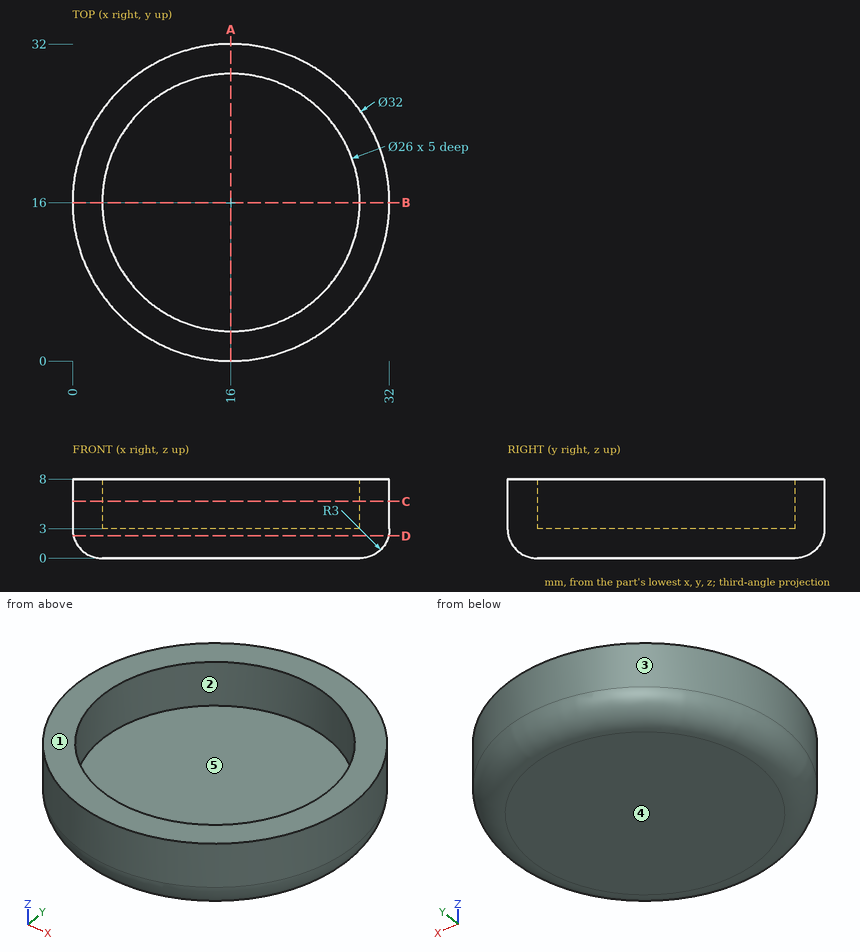
Job drawing, mm, ordinate dimensions from the low corner. One solid piece. A direction names the side the tool comes from. Give positions to 0.01 mm unless a question says otherwise; leave off trailing zeros. Loops run counter-clockwise (first coordinate to the right, second up) from the corner with the lowest first, then second, coordinate; pieces in that order, holes last. Notation, with made-up numbers: (-37, -31.5) -> (-22, -31.5) arc R5 ccw to (-22, -22.5) -> close; hole circle Ø5 at (4.5, 36). An arc over 180 degrees is marked (long way). Use a Markdown table: item, result. Add a question column.
(1) Wall check: line 1 along Y through (x, z) = (16, 4.85); line 2 along Z through (x, y) = (10.5, 22); line 3 along Y through (x, z) = (28, 6.25). Give the ranges that are in metal, low to high.
(2) Slice it at D-D on z = 2.25. List the corners of the cut face in (x, y).
(3) Slice it at A-A on x = 16. List the corners of the cut face in (y, z), and give its area (3 significant figures).
(4) Slice it at C-C on z = 5.75. List the corners of the cut face in (x, y).
(5) Drop flat-ended pins along their axis: pin 1 Ø4 at (x, z) = (7, 3) entering from -Y; pin 2 Ø1.5 at (x, z) = (5, 4) entering from +Y; pin 3 Ø1.5 at (y, z) = (11, 3.5) entering from -X. Give the stop position or say it passes through.
(6) Tool access for the marked faces 1 and 2: list every direction of +Z, -Z, +X, -X, +Y, -Y with a clear straight run to the whole face (end or side of a thin tool).
(7) Mould opens along X. For the marked faces 3, 4 and 5 say: +X half, -X half, draft (parallel to the pull), parting line (faces both ways), or undercut.
Filled sheet:
| question | item | result |
|---|---|---|
| 1 | line 1 | 0 to 3, 29 to 32 |
| 1 | line 2 | 0 to 3 |
| 1 | line 3 | 5.42 to 11, 21 to 26.58 |
| 2 | outline | circle Ø31.81 at (16, 16) |
| 3 | outline | (0, 3) arc R3 ccw to (3, 0) -> (29, 0) arc R3 ccw to (32, 3) -> (32, 8) -> (29, 8) -> (29, 3) -> (3, 3) -> (3, 8) -> (0, 8) -> close |
| 3 | area | 122 mm2 |
| 4 | outline | circle Ø32 at (16, 16); hole circle Ø26 at (16, 16) |
| 5 | pin 1 | y = 1.61 |
| 5 | pin 2 | y = 28.29 |
| 5 | pin 3 | x = 0.57 |
| 6 | face 1 | +Z, +X, -X, +Y, -Y |
| 6 | face 2 | +Z |
| 7 | face 3 | parting line |
| 7 | face 4 | draft |
| 7 | face 5 | undercut |
